Read the model definition and answer for the solid it produces. Units are mm, in the model's axes. Face numbers are marked on the shaded views. A direction names the side the tool comes from. Round coordinates to 2 decimals unless told otherwise and drop trailing zeros. Write each loop counter-clockwise with the first axis right and the second up, starting at its lowest first coordinate (ties: lowest second). Pieces come first, ordered by that corner, then holes.
from build123d import *

# Parameters (mm, degrees)
SKETCH3_OUTSIDE_W  = 11.216
SKETCH3_OUTSIDE_H  = 11.216
CUT_EXTRUDE1_DEPTH = 8


with BuildPart() as part:
    # Sketch1 → Revolve3 (revolve)
    with BuildSketch(Plane.XY):
        with BuildLine():
            ThreePointArc((1, 10), (1.994262201, 8.419337011), (1.25, 6.706699693))
            Line((1.25, 6.706699693), (1.25, 5.5))
            Line((1.25, 5.5), (0, 5.5))
            Line((0, 5.5), (0, 10))
            Line((0, 10), (1, 10))
        make_face()
        Polygon((0, 0), (0, 5.5), (1.25, 5.5), (3.25, 3.5), (3.25, 3), (1.5, 3), (1.5, 0), align=None)
    revolve(axis=Axis((0, 5.5, 0), (0, 1, 0)))

    # Sketch3 outside → Cut-Extrude1 (cut, through all)
    with BuildSketch(Plane.XZ.offset(-3)):
        Rectangle(SKETCH3_OUTSIDE_W, SKETCH3_OUTSIDE_H)
        Polygon((0, 3.25), (-2.814582562, 1.625), (-2.814582562, -1.625), (0, -3.25), (2.814582562, -1.625), (2.814582562, 1.625), align=None, mode=Mode.SUBTRACT)
    extrude(amount=-CUT_EXTRUDE1_DEPTH, mode=Mode.SUBTRACT)


solid = part.part
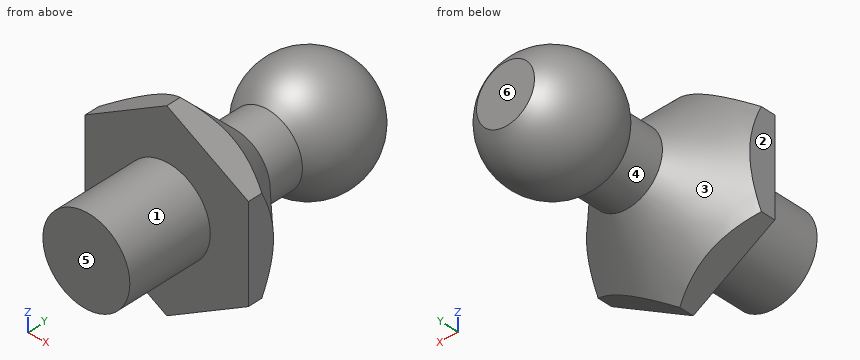
Q1. Section A-A (z = 0) is taken. Determine the outline of the cut face in (x, y).
Verdict:
outline: (-2.81, 3) - (-1.5, 3) - (-1.5, 0) - (1.5, 0) - (1.5, 3) - (2.81, 3) - (2.81, 3.94) - (1.25, 5.5) - (1.25, 6.71) arc R2 ccw to (1, 10) - (-1, 10) arc R2 ccw to (-1.25, 6.71) - (-1.25, 5.5) - (-2.81, 3.94) - close
Q2. Section D-D (y = 8.25) is taken. Determine the outline of the cut face in (x, z).
Verdict:
outline: circle Ø4 at (0, 0)
Q3. Flat-ended cylindrical pins translate along their axes: pin 1 Ø1 at (x, y) = (2, 3) entering from -Z; pin 2 Ø1.5 at (x, z) = (-1, -0.5) entering from -Y; pin 3 Ø2 at (y, z) = (9, 0.5) entering from -X. Find the tip coordinate at first contact, or state that the pin passes through.
Verdict:
pin 1: stops at z = -2.38
pin 2: stops at y = 0
pin 3: stops at x = -2
Q4. Section C-C (y = 2) is taken. Determine the outline of the cut face in (x, z).
Verdict:
outline: circle Ø3 at (0, 0)
Q5. Section B-B (y = 3.75) is taken. Determine the outline of the cut face in (x, z).
Verdict:
outline: (-2.81, -1.04) arc R3 ccw to (-2.31, -1.92) - (-0.51, -2.96) arc R3 ccw to (0.51, -2.96) - (2.31, -1.92) arc R3 ccw to (2.81, -1.04) - (2.81, 1.04) arc R3 ccw to (2.31, 1.92) - (0.51, 2.96) arc R3 ccw to (-0.51, 2.96) - (-2.31, 1.92) arc R3 ccw to (-2.81, 1.04) - close
Q6. Straight lines are drawn through the part: probe 1 along Y at (x, z) = (1.6, 0.75); probe 2 along Y at (x, z) = (1.55, -0.25); probe 3 along X at (y, z) = (6, 0). For each, find the intervals that lie inside material, in ascending order.
Verdict:
probe 1: y = 3 to 4.98, 7.33 to 9.2
probe 2: y = 3 to 5.18, 7.03 to 9.51
probe 3: x = -1.25 to 1.25
Q7. Which of the six approach directions +Z, -Z, +X, -X, +Y, -Y give full straight-line access (tool end or side, diameter ignored) to the marked faces 1 and 2?
Verdict:
face 1: -Y
face 2: +Z, -Z, -X, +Y, -Y
Q8. Determine the mould class of the marked faces 3, 4, 5 and 6 for opening direction Y: pulls with the +Y half, pulls with the -Y half, needs draft (parallel to the pull), parting line crosses it, or undercut.
Verdict:
face 3: undercut
face 4: undercut
face 5: pulls with the -Y half
face 6: pulls with the +Y half
